Model file for the job. Use its own axes, mm. Face numbers are marked on the shaded views. Round coordinates to 2 decimals unless told otherwise and drop trailing zeros. Loops run counter-clockwise (first coordinate to the right, second up) from the corner with the lowest first, then second, coordinate; pieces in that order, holes last. Notation, with made-up numbers: M 38,-33 L 75,-33 A29 ccw 75,-5 Z; hole C 15.5,17 d6. An arc over 180 degrees is marked long. Use a Markdown table: item, result. Add a question column.
Item 1: Saw through at A-A on x = 0. Write the cut outline in (y, z).
Item 2: Two-plate mould, pull along X, no slides. Class the marked faces 1, 2 and 3: +X half, -X half, draft (parallel to the pull), parting line (faces both ways), or undercut.
Item 3: Pin check, flat tips, straight feed: P1, Ø3, axis at y = 0.5, z = 3, coming from the -X side; P2, Ø2, axis at y = 1.5, z = -2, coming from the +X side; P3, Ø1.2, axis at x = 6, z = 0, coming from the +Y side. Stop position of each tip, or through.
Item 4: Saw through at B-B on z = 0. Write the cut outline in (x, y), then the cut area to 3 significant figures.
Item 5: Saw through at C-C on y = 2.2. Write the cut outline in (x, z), then the cut area to 3 significant figures.
Item 6: Wall check: L1, parallel to X at y = 3.75, z = 0; L2, parallel to X at y = 2.4, z = 1. Give the ranges that are in metal, low to high. Write a range as from..to.
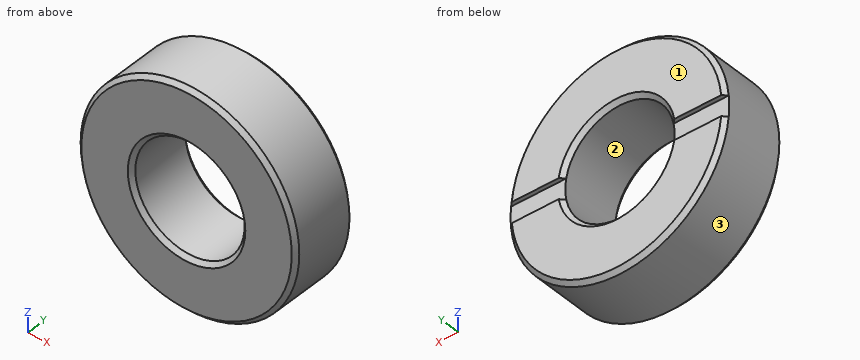
Autodesk Inventor part; units mm, degrees
ref_plane "YZ Plane" through (0, 0, 0) normal (1, 0, 0) x (0, 1, 0)
ref_plane "XZ Plane" through (0, 0, 0) normal (0, 1, 0) x (-1, 0, 0)
ref_plane "XY Plane" through (0, 0, 0) normal (0, 0, 1) x (1, 0, 0)
sketch "スケッチ1" plane through (0, 0, 0) normal (0, 1, 0) x (-1, 0, 0)
  circle A0 centre (0, 0) radius 8
  circle A1 centre (0, 0) radius 4
  dimension "d0" = 16
  dimension "d1" = 8
extrude "押し出し1" add sketch "スケッチ1" along normal blind 5
sketch "スケッチ2" plane through (0, 5, 0) normal (0, 1, 0) x (1, 0, 0)
  circle A0 centre (0, 0) radius 8
  line L0 (-8, 0) -> (8, 0)
  line L1 (-8, 0.75) -> (8, 0.75)
  line L2 (-8, 0.75) -> (-8, 0)
  line L3 (8, 0.75) -> (8, 0)
  line L4 (-8, -0.75) -> (8, -0.75)
  line L5 (-8, -0.75) -> (-8, 0)
  line L6 (8, -0.75) -> (8, 0)
  point P0 (7.9648, 0.75)
  point P1 (-7.9648, 0.75)
  point P2 (-7.9648, -0.75)
  point P3 (7.9648, -0.75)
  dimension "d4" = 0.75
extrude "押し出し2" cut sketch "スケッチ2" against normal blind 0.3 contours L0 A0 L1 | A0 L4 L0
chamfer "面取り1" distance 0.3 angle 45 6 edges at (0, 5, 4) (0, 5, -4) (0, 5, -8) (0, 5, 8) (8, 0, 0) (4, 0, 0)
properties part number "GSB-081605"
Entries:
| question | item | result |
|---|---|---|
| 1 | outline | M 0,-7.7 L 0.3,-8 L 4.7,-8 L 5,-7.7 L 5,-4.3 L 4.7,-4 L 0.3,-4 L 0,-4.3 Z; M 0,4.3 L 0.3,4 L 4.7,4 L 5,4.3 L 5,7.7 L 4.7,8 L 0.3,8 L 0,7.7 Z |
| 2 | face 1 | draft |
| 2 | face 2 | undercut |
| 2 | face 3 | parting line |
| 3 | P1 | x = -7.86 |
| 3 | P2 | x = 7.94 |
| 3 | P3 | y = 4.7 |
| 4 | outline | M -8,0.3 L -7.7,0 L -4.3,0 L -4,0.3 L -4,4.7 L -8,4.7 Z; M 4,0.3 L 4.3,0 L 7.7,0 L 8,0.3 L 8,4.7 L 4,4.7 Z |
| 4 | area | 37.4 mm2 |
| 5 | outline | C 0,0 d16; hole C 0,0 d8 |
| 5 | area | 151 mm2 |
| 6 | L1 | -8..-4, 4..8 |
| 6 | L2 | -7.94..-3.87, 3.87..7.94 |
